from build123d import *

# Parameters (mm, degrees)
SALIENTE_EXTRUIR1_DEPTH = 3
CROQUIS2_W              = 3
CROQUIS2_H              = 10
CROQUIS2_W_2            = 20
CROQUIS2_H_2            = 3
SALIENTE_EXTRUIR2_DEPTH = 3


with BuildPart() as part:
    # Croquis1 → Saliente-Extruir1 (new body)
    with BuildSketch(Plane.XY):
        Polygon((18, -3), (57, -3), (57, -31.8), (72, -31.8), (72, -60.3), (3, -60.3), (3, -31.8), (18, -31.8), align=None)
    extrude(amount=SALIENTE_EXTRUIR1_DEPTH)

    # Croquis2 → Saliente-Extruir2 (add)
    with BuildSketch(Plane.XY.offset(3)):
        with Locations((73.5, -46.05)):
            Rectangle(CROQUIS2_W, CROQUIS2_H)
        with Locations((1.5, -46.05)):
            Rectangle(CROQUIS2_W, CROQUIS2_H)
        with Locations((37.5, -1.5)):
            Rectangle(CROQUIS2_W_2, CROQUIS2_H_2)
    extrude(amount=-SALIENTE_EXTRUIR2_DEPTH)


solid = part.part
Geometry: final body of the model. Coordinates: model frame, mm. A direction names the side the tool comes from. Give positions to 0.01 mm unless a question says otherwise; leave off trailing zeros. Write each loop counter-clockwise with the first axis right and the second up, starting at its lowest first coordinate (ties: lowest second). Pieces come first, ordered by that corner, then holes.
(1) Cut plane B-B, the plane x = 6. Return loops of the section in (y, z).
(2) Cut plane C-C, the plane y = -30. Return loops of the section in (x, z).
(3) Ray query, line 1 (Y direction, x = 58, z = 0.45); line 2 (X direction, y = -14, z = 2); line 3 (Y direction, x = 27, z = 1.15). Return the intervals inside material, ascending.
(4) Access query for faces 4 (the flat face through (1, -51.05, 2)), 5 (the flat face through (52, -3, 1)), 6 (the flat face through (72, -56, 1)), 7 (the flat face through (18, -18, 1)). Directions: +Z, -Z, +X, -X, +Y, -Y. A direction counts if a zero-diameter tool reaches every point of the face in a straight line with its end or side. Return the directions, or none.
(5) First-contact query: P1, Ø1.5, axis at y = -36, z = 1, coming from the +X side; P2, Ø0.9, axis at x = 2, z = 1.5, coming from the -Y side; P3, Ø1.5, axis at x = 22, z = 1.5, coming from the +Y side. Flat tips, straight axial feed; report the tip coordinate or a pass-through.
(6) Mould query, pull axis Z, two halves, no side actions, for faces 1 (the flat face through (38, -36, 3)), 2 (the flat face through (73, -41.05, 2)), 3 (the flat face through (38, -36, 0)). Classes: released by +Z, released by -Z, zero draft, split by the parting line, or undercut.
(7) Cut plane A-A, the plane z = 0.9. Return loops of the section in (x, y).
Values follow:
1. outline: (-60.3, 0) - (-31.8, 0) - (-31.8, 3) - (-60.3, 3) - close
2. outline: (18, 0) - (57, 0) - (57, 3) - (18, 3) - close
3. line 1: y = -60.3 to -31.8
3. line 2: x = 18 to 57
3. line 3: y = -60.3 to -3
4. face 4: +Z, -Z, -X, -Y
4. face 5: +Z, -Z, +X, +Y
4. face 6: +Z, -Z, +X, -Y
4. face 7: +Z, -Z, -X, +Y
5. P1: stops at x = 72
5. P2: stops at y = -51.05
5. P3: stops at y = -3
6. face 1: released by +Z
6. face 2: zero draft
6. face 3: released by -Z
7. outline: (0, -51.05) - (3, -51.05) - (3, -60.3) - (72, -60.3) - (72, -51.05) - (75, -51.05) - (75, -41.05) - (72, -41.05) - (72, -31.8) - (57, -31.8) - (57, -3) - (47.5, -3) - (47.5, 0) - (27.5, 0) - (27.5, -3) - (18, -3) - (18, -31.8) - (3, -31.8) - (3, -41.05) - (0, -41.05) - close
